Here's the drawing with two shaded views (mm, measured from the low corner). I have some questions. Round coordinates to 2 decimals unless told otherwise and drop trailing zeros. Loops run counter-clockwise (first coordinate to the right, second up) from the corner with the lowest first, then second, coordinate; pieces in that order, holes last.
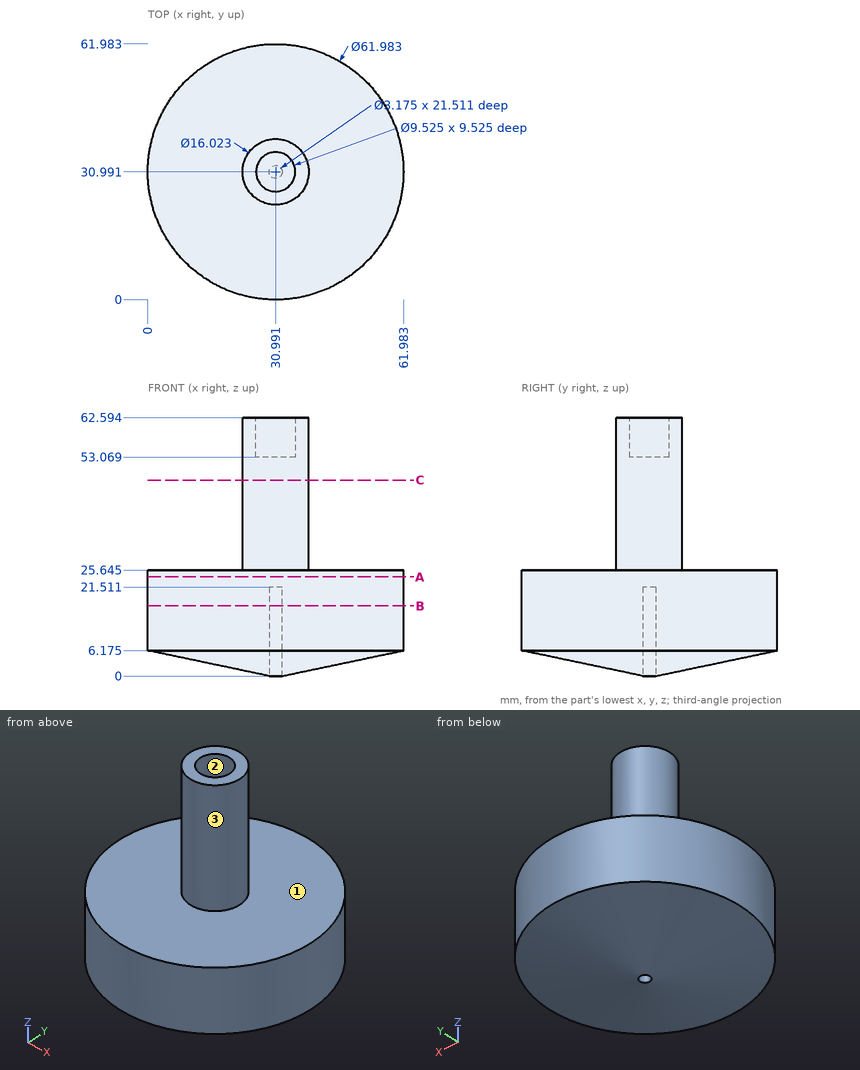
(1) If I drill on line 1 (Y direction, x = 30.5, z = 15.5) (1 decimal); line 2 (Z direction, x = 21, y = 24) (1 decimal); line 3 (Z direction, x = 15.5, y = 5.5) (1 decimal), over which ranges is the centre line in solid material (lowest first)?
Worked answers:
line 1: y = 0 to 29.5, 32.5 to 62
line 2: z = 2.2 to 25.6
line 3: z = 5.9 to 25.6
(2) Will these pins go through, and if not, where does the flat tip stop? P1, Ø5, axis at y = 16.5, z = 22.5, coming from the +X side; P2, Ø3, axis at x = 13.5, z = 18.5, coming from the +Y side; P3, Ø8, axis at y = 9.5, z = 16.5, coming from the -X side.
Worked answers:
P1: stops at x = 59.57
P2: stops at y = 57.54
P3: stops at x = 5.41
(3) If we mould it in two halves opening along X, with no side actions, what happens to the marked faces 1, 2 and 3? For each: released by +X, released by -X, zero draft, split by the parting line, or undercut.
Worked answers:
face 1: zero draft
face 2: undercut
face 3: split by the parting line
(4) If we section it at B-B, the plane z = 17: List the corners of the cut face in (x, y) for me (1 decimal).
Worked answers:
outline: circle Ø62 at (31, 31); hole circle Ø3.2 at (31, 31)
(5) If we section it at A-A, the plane z = 24: List the corners of the cut face in (x, y) for me, then the cut area to 3 significant figures.
Worked answers:
outline: circle Ø61.98 at (30.99, 30.99)
area: 3,020 mm2
(6) If we section it at C-C, the plane z = 47.5: List the corners of the cut face in (x, y) for me, then the cut area to 3 significant figures.
Worked answers:
outline: circle Ø16.02 at (30.99, 30.99)
area: 202 mm2
